Verification items for the finished model (mm, model axes). Round coordinates to 2 decimals unless told otherwise and drop trailing zeros. Loops run counter-clockwise (first coordinate to the right, second up) from the corner with the lowest first, then second, coordinate; pieces in that order, holes last. Notation, with made-up numbers: M -17,-27.75 L 24,-27.75 A21 ccw 24,0.25 Z; hole C 38.5,32.5 d1. An arc over 180 degrees is marked long. Answer as CSV lines item,"result".
```python
from build123d import *

# Parameters (mm, degrees)
SKETCH1_R           = 4
SKETCH1_R_2         = 4.5
BOSS_EXTRUDE1_DEPTH = 2
CHAMFER1_SIZE       = 2
CHAMFER2_SIZE       = 10


with BuildPart() as part:
    # Sketch1 → Boss-Extrude1 (new body)
    with BuildSketch(Plane(origin=(0, 0, 0), x_dir=(1, 0, 0), z_dir=(0, 1, 0))):
        with BuildLine():
            Line((0, 0), (245, 0))
            Line((245, 0), (245, 15))
            ThreePointArc((245, 15), (241, 32.5), (245, 50))
            Line((245, 50), (245, 255))
            Line((245, 255), (0, 255))
            Line((0, 255), (0, 50))
            ThreePointArc((0, 50), (4, 32.5), (0, 15))
            Line((0, 15), (0, 0))
        make_face()
        with Locations(Location((8, 7, 0), (0, 0, 270))):
            Circle(SKETCH1_R, mode=Mode.SUBTRACT)
        with Locations(Location((22, 7, 0), (0, 0, 270))):
            Circle(SKETCH1_R, mode=Mode.SUBTRACT)
        with Locations(Location((237, 7, 0), (0, 0, 270))):
            Circle(SKETCH1_R, mode=Mode.SUBTRACT)
        with Locations(Location((223, 7, 0), (0, 0, 270))):
            Circle(SKETCH1_R, mode=Mode.SUBTRACT)
        with Locations(Location((27, 27, 0), (0, 0, 270))):
            Circle(SKETCH1_R_2, mode=Mode.SUBTRACT)
        with Locations(Location((82, 27, 0), (0, 0, 270))):
            Circle(SKETCH1_R_2, mode=Mode.SUBTRACT)
        with Locations(Location((162, 27, 0), (0, 0, 270))):
            Circle(SKETCH1_R_2, mode=Mode.SUBTRACT)
        with Locations(Location((217, 27, 0), (0, 0, 270))):
            Circle(SKETCH1_R_2, mode=Mode.SUBTRACT)
        with Locations(Location((27, 127, 0), (0, 0, 270))):
            Circle(SKETCH1_R_2, mode=Mode.SUBTRACT)
        with Locations(Location((92, 127, 0), (0, 0, 270))):
            Circle(SKETCH1_R_2, mode=Mode.SUBTRACT)
        with Locations(Location((152, 127, 0), (0, 0, 270))):
            Circle(SKETCH1_R_2, mode=Mode.SUBTRACT)
        with Locations(Location((217, 127, 0), (0, 0, 270))):
            Circle(SKETCH1_R_2, mode=Mode.SUBTRACT)
        with Locations(Location((27, 230, 0), (0, 0, 270))):
            Circle(SKETCH1_R_2, mode=Mode.SUBTRACT)
        with Locations(Location((147, 230, 0), (0, 0, 270))):
            Circle(SKETCH1_R_2, mode=Mode.SUBTRACT)
        with Locations(Location((216, 230, 0), (0, 0, 270))):
            Circle(SKETCH1_R_2, mode=Mode.SUBTRACT)
        with Locations(Location((54, 247, 0), (0, 0, 270))):
            Circle(SKETCH1_R, mode=Mode.SUBTRACT)
        with Locations(Location((66.5, 247, 0), (0, 0, 270))):
            Circle(SKETCH1_R, mode=Mode.SUBTRACT)
        with Locations(Location((179.5, 247, 0), (0, 0, 270))):
            Circle(SKETCH1_R, mode=Mode.SUBTRACT)
        with Locations(Location((192, 247, 0), (0, 0, 270))):
            Circle(SKETCH1_R, mode=Mode.SUBTRACT)
    extrude(amount=BOSS_EXTRUDE1_DEPTH)

    # Chamfer1
    chamfer1_edges = [part.edges().sort_by_distance(p)[0] for p in [
        (245, 1, 0),
        (0, 1, 0),
    ]]
    chamfer(chamfer1_edges, length=CHAMFER1_SIZE)

    # Chamfer2
    chamfer2_edges = [part.edges().sort_by_distance(p)[0] for p in [
        (0, 1, -255),
        (245, 1, -255),
    ]]
    chamfer(chamfer2_edges, length=CHAMFER2_SIZE)


solid = part.part
```
1) Material ranges on probe 1 along X at (y, z) = (0.4, -127); probe 2 along X at (y, z) = (1.1, -7); probe 3 along Z at (x, y) = (64.5, 1.85), recorded low to high.
Here are the results:
probe 1,"x = 0 to 22.5, 31.5 to 87.5, 96.5 to 147.5, 156.5 to 212.5, 221.5 to 245"
probe 2,"x = 0 to 4, 12 to 18, 26 to 219, 227 to 233, 241 to 245"
probe 3,"z = -255 to -250.46, -243.54 to 0"
2) Section check C-C (y = 0.45). State how many separate pieces and enclosed holes the cut face has, plus the area to 3 significant figures.
Here are the results:
separate pieces,"1"
enclosed holes,"19"
area,"61,100 mm^2"
3) Draft check along Z on faces 1 (the flat face through (121, 2, -129)), 2 (the cylindrical face through (86.46, 0.99, -27.59)), 3 (the flat face through (5, 1, -250)). Enter one of: +Z half, -Z half, draft (parallel to the pull), parting line (faces both ways), or undercut.
Here are the results:
face 1,"draft"
face 2,"undercut"
face 3,"-Z half"
4) Section check B-B (x = 54). Record the cut outline in (y, z).
Here are the results:
outline,"M 0,-255 L 2,-255 L 2,-251 L 0,-251 Z; M 0,-243 L 2,-243 L 2,0 L 0,0 Z"
5) Section check D-D (x = 92). Record the cut outline in (y, z).
Here are the results:
outline,"M 0,-255 L 2,-255 L 2,-131.5 L 0,-131.5 Z; M 0,-122.5 L 2,-122.5 L 2,0 L 0,0 Z"
6) Section check A-A (z = -127). Record the cut outline in (x, y).
Here are the results:
outline,"M 0,0 L 22.5,0 L 22.5,2 L 0,2 Z; M 31.5,0 L 87.5,0 L 87.5,2 L 31.5,2 Z; M 96.5,0 L 147.5,0 L 147.5,2 L 96.5,2 Z; M 156.5,0 L 212.5,0 L 212.5,2 L 156.5,2 Z; M 221.5,0 L 245,0 L 245,2 L 221.5,2 Z"
